Geometry: see drawing. Coordinates: mm, zero at the bounding-box minimum. A direction names the side the tool comes from. Coordinates: 2 decimals unless noted, no trailing zeros. Order: outer loops, then holes, each group sorted by start corner. A loop starts at its lowest first (then second) coordinate and runs counter-clockwise, first axis right, second up. Notation, with made-up numbers: M 22,87 L 34,87 A13 ccw 34,108 Z; hole C 83,-38 d2. An arc over 180 degrees is marked long. One line per item, written item: value.
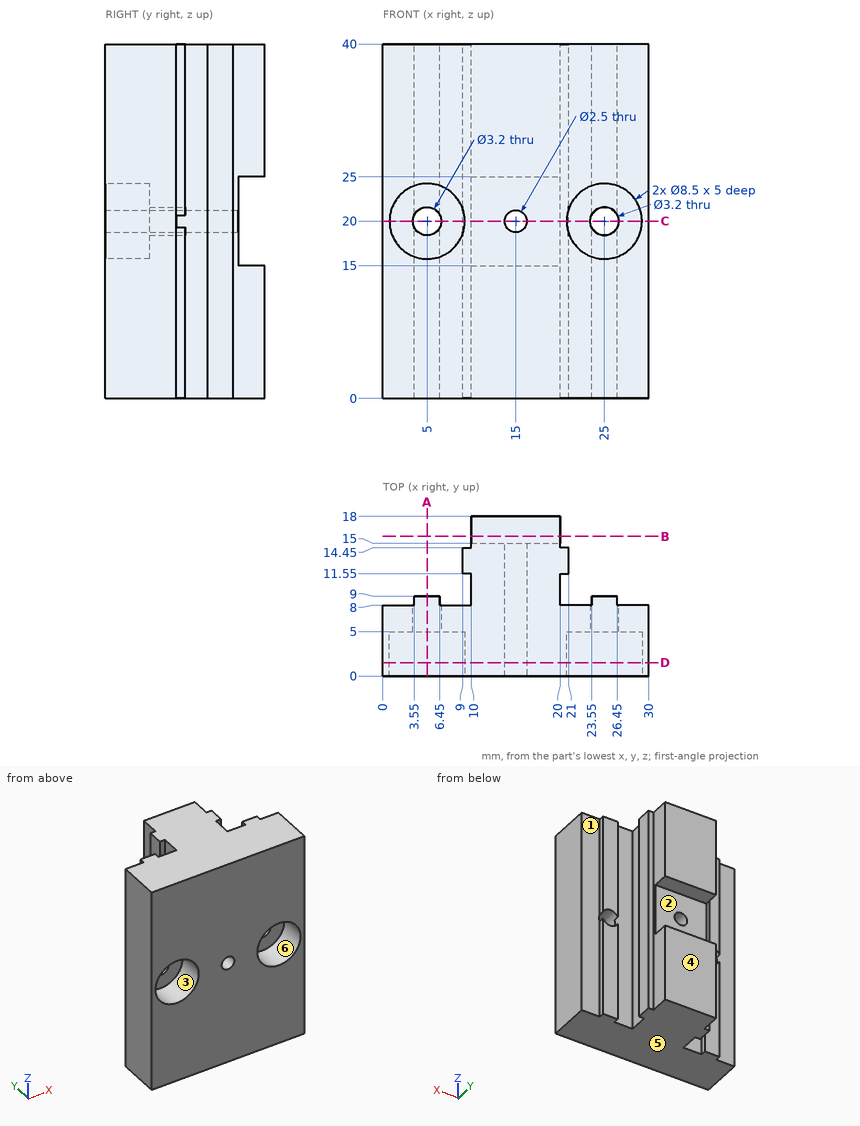
(1) Draft query along Z for the marked faces 4, 5 and 6. Return one class per face: released by +Z, released by -Z, zero draft, split by the parting line, or undercut.
Data:
face 4: zero draft
face 5: released by -Z
face 6: undercut
(2) Cut plane B-B on y = 15.75. Output: boundary loops of the cut face in (x, z), plus the area to 3 significant figures.
Data:
outline: M 10,0 L 20,0 L 20,15 L 10,15 Z; M 10,25 L 20,25 L 20,40 L 10,40 Z
area: 300 mm2
(3) Cut plane D-D on y = 1.5. Output: boundary loops of the cut face in (x, z).
Data:
outline: M 0,0 L 30,0 L 30,40 L 0,40 Z; hole C 5,20 d8.5; hole C 15,20 d2.5; hole C 25,20 d8.5
(4) Cut plane A-A on x = 5. Output: boundary loops of the cut face in (y, z), plus the area to 3 significant figures.
Data:
outline: M 0,0 L 9,0 L 9,18.4 L 5,18.4 L 5,15.75 L 0,15.75 Z; M 0,24.25 L 5,24.25 L 5,21.6 L 9,21.6 L 9,40 L 0,40 Z
area: 305 mm2
(5) Ray query, line 1 (X direction, y = 1.9, z = 20); line 2 (Z direction, x = 25, y = 1.2); line 3 (Y direction, x = 20.75, z = 28.5). Return the intervals inside material, ascending. Write a range as from..to.
Data:
line 1: x = 0..0.75, 9.25..13.75, 16.25..20.75, 29.25..30
line 2: z = 0..15.75, 24.25..40
line 3: y = 0..8, 11.55..14.45
(6) First-contact query: pin 1 (0.9 mm diameter, centred on y = 13.5, z = 26, fed in from +X); pin 2 (3 mm diameter, centred on x = 17, z = 20.5, fed in from +Y); pin 3 (5 mm diameter, centred on x = 5, z = 20, fed in from +Y). Flat tips, straight axial feed; report the tip coordinate or a pass-through.
Data:
pin 1: stops at x = 21
pin 2: stops at y = 15
pin 3: stops at y = 9
(7) Access query for the marked faces 1, 2 and 3. Directions: +Z, -Z, +X, -X, +Y, -Y. A direction counts if a zero-diameter tool reaches every point of the face in a straight line with its end or side. Return the directions, or none.
Data:
face 1: +Z, -Z, +X, +Y
face 2: +X, -X, +Y
face 3: -Y
(8) Cut plane C-C on z = 20. Give the number of separate pieces and of enclosed holes in the cut face, plus the area to 3 significant figures.
Data:
separate pieces: 4
enclosed holes: 0
area: 174 mm2
